Geometry check sheet. Reference: drawing and pictorial views, mm from the part's lowest x, y, z. A direction names the side the tool comes from. Give positions to 0.01 mm unless a question says otherwise; leave off trailing zeros. Write each loop counter-clockwise with the first axis right and the second up, starting at its lowest first coordinate (ties: lowest second). Pieces come first, ordered by that corner, then holes. Notation, with made-up numbers: (5, 76.25) - (22, 76.25) arc R14 cw to (22, 93.25) - close; hole circle Ø7 at (72.5, 54.5). An arc over 180 degrees is marked (long way). Write item = value, one per line. Start each with the question number.
(1) Section check B-B, the plane z = 18.5. Enter the section's corners in (x, y).
(2) Depth check by flat-ended pin: pin 1 Ø1.8 at (x, z) = (13.5, 7.5) entering from -Y; pin 2 Ø2 at (x, y) = (18, 2.5) entering from +Z; pin 3 Ø1.4 at (x, z) = (14.5, 12.5) entering from -Y; pin 4 Ø3 at (y, z) = (1.5, 9.5) entering from -X. Enter the tip coordinate at first touch or a pass-through.
(3) Draft check along X on the marked faces 3, 4, 5 and 6. Enter one of: pulls with the +X half, pulls with the -X half, needs draft (parallel to the pull), parting line crosses it, or undercut.
(4) Section check D-D, the plane z = 5. Enter the section's corners in (x, y).
(5) Section check A-A, the plane x = 13.5. Enter the section's corners in (y, z).
(6) Thickness scan on L1, parallel to Z at x = 13.5, y = 1.65; L2, parallel to Z at x = 13.5, y = 3.25; L3, parallel to X at y = 1.7, z = 13.5. Record the ranges inside material, lowest first.
(7) Access from +Z, -Z, +X, -X, +Y, -Y to the whole of each face (thin tool, end or side, straight path). Record for the marked faces 1 and 2.
(8) Section check C-C, the plane y = 4.1. Enter the section's corners in (x, z).
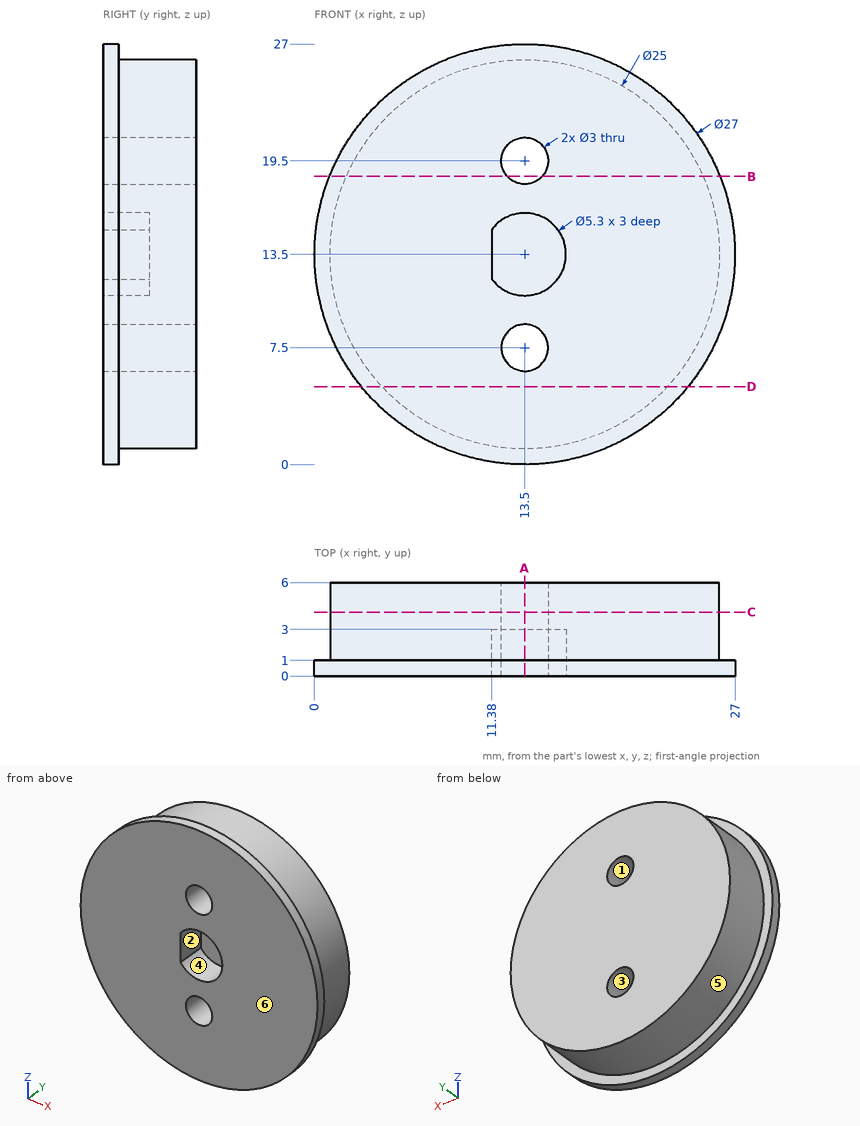
Model answer:
q1.outline = (0.96, 0) - (12.38, 0) - (12.38, 6) - (2.04, 6) - (2.04, 1) - (0.96, 1) - close; (14.62, 0) - (26.04, 0) - (26.04, 1) - (24.96, 1) - (24.96, 6) - (14.62, 6) - close
q2.pin_1 = through
q2.pin_2 = 25.5
q2.pin_3 = 3
q2.pin_4 = 0.25
q3.face_3 = undercut
q3.face_4 = undercut
q3.face_5 = parting line crosses it
q3.face_6 = needs draft
q4.outline = (3.01, 0) - (23.99, 0) - (23.99, 1) - (22.67, 1) - (22.67, 6) - (4.33, 6) - (4.33, 1) - (3.01, 1) - close
q5.outline = (0, 0) - (1, 0) - (1, 1) - (6, 1) - (6, 6) - (0, 6) - close; (0, 9) - (6, 9) - (6, 18) - (0, 18) - (0, 16.15) - (3, 16.15) - (3, 10.85) - (0, 10.85) - close; (0, 21) - (6, 21) - (6, 26) - (1, 26) - (1, 27) - (0, 27) - close
q6.L1 = 1 to 6, 9 to 10.85, 16.15 to 18, 21 to 26
q6.L2 = 1 to 6, 9 to 18, 21 to 26
q6.L3 = 1 to 11.38, 16.15 to 26
q7.face_1 = +Y, -Y
q7.face_2 = -Y
q8.outline = circle Ø25 at (13.5, 13.5); hole circle Ø3 at (13.5, 7.5); hole circle Ø3 at (13.5, 19.5)
